Check sheet for the modelled part. Datum: model origin and axes. Units: mm. A direction names the side the tool comes from. Round coordinates to 2 decimals unless told otherwise and drop trailing zeros. Order: outer loops, then holes, each group sorted by start corner. A loop starts at its lowest first (then second) coordinate and runs counter-clockwise, first axis right, second up.
(1) Depth check by flat-ended pin: pin 1 (4 mm diameter, centred on x = 5.5, z = 29, fed in from +Y); pin 2 (3 mm diameter, centred on y = 22, z = 28.5, fed in from -X); pin 3 (8 mm diameter, centred on x = 6, y = -5, fed in from +Z); pin 4 (2 mm diameter, centred on x = 5, z = -29, fed in from -Y). Enter the tip coordinate at first touch or a pass-through.
(2) Sectioned sample at A-A, the plane z = 0. Enter the section's corners in (x, y).
(3) Thickness scan on probe 1 along Y at (x, z) = (17.85, 0); probe 2 along Z at (x, y) = (15.5, 0). Record the ranges inside material, lowest first.
(4) Sectioned sample at C-C, the plane x = 8.5. Enter the section's corners in (y, z).
(5) Tool access check on faces 5 (the flat face through (0, -1, -1)), 6 (the flat face through (16, -20, -5)), 7 (the cylindrical face through (8.465, -1.055, -23.977)). Record the directions out of +Z, -Z, +X, -X, +Y, -Y that give a thin tool (end or side, any length) a straight path to the whole face; none if there is none.
(6) Mould release check, pull along Y, two halves, no side actions. Record for faces 1 (the cylindrical face through (13.465, 19.524, -4.336)), 2 (the flat face through (11, -20, 5)), 3 (the cylindrical face through (16.04, -0.53, -11.99)), 4 (the flat face through (10, 0, 0)): released by +Y, released by -Y, zero draft, split by the parting line, or undercut.
```python
from build123d import *

# Parameters (mm, degrees)
F2_SIZE = 1
F3_R    = 3


with BuildPart() as f1:
    # F0 (on Front) → F1 (revolve)
    with BuildSketch(Plane.XZ):
        Polygon((0, 40), (0, 0), (10, 0), (10, 12), (19, 12), (19, 24), (16, 24), (16, 20), (11, 20), (11, 24), (6, 24), (6, 40), align=None)
    revolve(axis=Axis((9.5, 0, 0), (1, 0, 0)))

    # F2
    f2_edges = [f1.edges().sort_by_distance(p)[0] for p in [
        (0, 0, -40),
    ]]
    chamfer(f2_edges, length=F2_SIZE)

    # F3
    f3_edges = [f1.edges().sort_by_distance(p)[0] for p in [
        (10, 0, -12),
    ]]
    fillet(f3_edges, radius=F3_R)


solid = f1.part
```
Derived:
1. pin 1: stops at y = 29.51
1. pin 2: stops at x = 0
1. pin 3: stops at z = 39.99
1. pin 4: stops at y = -28.57
2. outline: (0, -39) - (1, -40) - (6, -40) - (6, -24) - (11, -24) - (11, -20) - (16, -20) - (16, -24) - (19, -24) - (19, -12) - (13, -12) arc R3 cw to (10, -9) - (10, 9) arc R3 cw to (13, 12) - (19, 12) - (19, 24) - (16, 24) - (16, 20) - (11, 20) - (11, 24) - (6, 24) - (6, 40) - (1, 40) - (0, 39) - close
3. probe 1: y = -24 to -12, 12 to 24
3. probe 2: z = -20 to -12, 12 to 20
4. outline: circle Ø48 at (0, 0)
5. face 5: +Z, -Z, -X, +Y, -Y
5. face 6: none
5. face 7: +X
6. face 1: split by the parting line
6. face 2: zero draft
6. face 3: undercut
6. face 4: undercut
